Here's how the part is built. I have some questions about the finished solid (model axes, mm). A direction names the side the tool comes from. Give positions to 0.01 mm unless a question says otherwise; leave off trailing zeros. Write each loop counter-clockwise with the first axis right and the second up, starting at its lowest first coordinate (ties: lowest second). Pieces come first, ordered by that corner, then holes. Notation, with made-up numbers: M -37.5,-11.5 L 11.5,-11.5 A15 cw 11.5,-7.5 Z; hole C 89.5,-20.5 d3. An arc over 180 degrees is marked long. Answer as CSV lines item,"result". Start each with the question number.
Q1. For pin 1 (10 mm diameter, centred on x = -1.5, y = 87.5, fed in from +Z); pin 2 (3 mm diameter, centred on x = 29, y = 5.5, fed in from -Z); pin 3 (1.5 mm diameter, centred on x = 7, z = 7.5, fed in from +Y); pin 4 (7.5 mm diameter, centred on y = 43.18, z = 0, fed in from -X), each with a flat end and sliding along its axis, tell me the tip position at first contact or that it passes through.
Q2. Suppose I cut it at B-B (y = 2.5). Write out the boundary of the cut face in (x, z) (3 decimals).
Q3. Thinking about a two-plate mould opening in Z: for faces 1 (the flat face through (-0.812, 56.483, -47.105)), 2 (the cylindrical face through (35.377, 5.151, -7.229)), 3 (the flat face through (-4.318, 60, -50)), which applies, +Z half, -Z half, draft (parallel to the pull), parting line (faces both ways), or undercut?
Q4. Suppose I cut it at A-A (z = 0). Write out the boundary of the cut face in (x, y) (3 decimals), then the cut area to 3 significant figures.
Q5. Suppose I cut it at D-D (z = -33). Write out the boundary of the cut face in (x, y) (3 decimals), then the cut area to 3 significant figures.
Q6. On a 3-axis mill with a long thin cutter (end or side, diameter ignored), from which of +Z, -Z, +X, -X, +Y, -Y can I reach the whole of each face in a straight line? I mean faces 4 (the flat face through (9.906, 42, 38)), 5 (the flat face through (-1, 79, 19.05)), 6 (the flat face through (6, 43, 19.05)), 7 (the flat face through (-0.812, 56.483, 47.105)). Say none if no direction works.
Q7. If I drill on line 1 along X through (y, z) = (-0.5, -42.5); line 2 along X through (y, z) = (58, -47.5); line 3 along Z through (x, y) = (-7, 76.5), over which ranges is the centre line in solid material (lowest first)?
Q8. Suppose I cut it at C-C (x = 0). Write out the boundary of the cut face in (y, z) (3 decimals).
```python
from build123d import *
from build123d.topology import SkipClean

# Parameters (mm, degrees)
SKETCH1_R           = 15.875
SKETCH1_R_2         = 6.35
BOSS_EXTRUDE1_DEPTH = 19.05
BOSS_EXTRUDE2_START = 19.05
SKETCH1_3_R         = 15.875
SKETCH1_3_R_2       = 6.35
BOSS_EXTRUDE2_DEPTH = 38.1
BOSS_EXTRUDE3_START = -19.05
SKETCH1_4_R         = 15.875
SKETCH1_4_R_2       = 6.35
BOSS_EXTRUDE3_DEPTH = 38.1
SKETCH2_W           = 7.112
SKETCH2_H           = 19.812
CUT_EXTRUDE1_DEPTH  = 138.602767
SKETCH4_R           = 6.35
SKETCH4_R_2         = 4.064
CUT_EXTRUDE2_DEPTH  = 123.816814
SKETCH5_R           = 3.175
SKETCH5_R_2         = 5.08
CUT_EXTRUDE3_DEPTH  = 117.109121


with BuildPart() as part:
    # Sketch1 → Boss-Extrude1 (new, symmetric)
    with BuildSketch(Plane.XY):
        Polygon((2.794, 97.536), (-9.906, 72.136), (0, 72.136), (2.794, 72.136), align=None)
        with BuildLine():
            Line((-9.906, 72.136), (-9.906, 12.405111))
            ThreePointArc((-9.906, 12.405111), (-5.24807, 14.982436), (0, 15.875))
            Line((0, 15.875), (0, 72.136))
            Line((0, 72.136), (-9.906, 72.136))
        make_face()
        with BuildLine():
            Line((0, 72.136), (0, 15.875))
            ThreePointArc((0, 15.875), (1.402484, 15.812927), (2.794, 15.627194))
            Line((2.794, 15.627194), (2.794, 72.136))
            Line((2.794, 72.136), (0, 72.136))
        make_face()
        Circle(SKETCH1_R)
        with Locations(Location((0, 0, 0), (0, 0, 180))):
            Circle(SKETCH1_R_2, mode=Mode.SUBTRACT)
        with BuildLine():
            ThreePointArc((12.197952, 10.16), (14.92746, 5.40246), (15.875, 0))
            Line((15.875, 0), (50.8, 0))
            Line((50.8, 0), (50.8, 10.16))
            Line((50.8, 10.16), (12.197952, 10.16))
        make_face()
    extrude(amount=BOSS_EXTRUDE1_DEPTH, both=True)

    # Sketch1<3> → Boss-Extrude2 (add)
    with BuildSketch(Plane.XY.offset(BOSS_EXTRUDE2_START)):
        with BuildLine():
            Line((-9.906, 72.136), (-9.906, 12.405111))
            ThreePointArc((-9.906, 12.405111), (-5.24807, 14.982436), (0, 15.875))
            Line((0, 15.875), (0, 72.136))
            Line((0, 72.136), (-9.906, 72.136))
        make_face()
        Circle(SKETCH1_3_R)
        with Locations(Location((0, 0, 0), (0, 0, 180))):
            Circle(SKETCH1_3_R_2, mode=Mode.SUBTRACT)
        with BuildLine():
            ThreePointArc((2.794, 15.627194), (6.55118, 14.46021), (9.906, 12.405111))
            Line((9.906, 12.405111), (9.906, 72.136))
            Line((9.906, 72.136), (2.794, 72.136))
            Line((2.794, 72.136), (2.794, 15.627194))
        make_face()
        with BuildLine():
            Line((0, 72.136), (0, 15.875))
            ThreePointArc((0, 15.875), (1.402484, 15.812927), (2.794, 15.627194))
            Line((2.794, 15.627194), (2.794, 72.136))
            Line((2.794, 72.136), (0, 72.136))
        make_face()
    extrude(amount=BOSS_EXTRUDE2_DEPTH)

    # Sketch1<4> → Boss-Extrude3 (add)
    with SkipClean():  # the faces are left unmerged after this step: merging them gives an invalid solid
        with BuildSketch(Plane.XY.offset(BOSS_EXTRUDE3_START)):
            with BuildLine():
                ThreePointArc((2.794, 15.627194), (6.55118, 14.46021), (9.906, 12.405111))
                Line((9.906, 12.405111), (9.906, 72.136))
                Line((9.906, 72.136), (2.794, 72.136))
                Line((2.794, 72.136), (2.794, 15.627194))
            make_face()
            with BuildLine():
                Line((-9.906, 72.136), (-9.906, 12.405111))
                ThreePointArc((-9.906, 12.405111), (-5.24807, 14.982436), (0, 15.875))
                Line((0, 15.875), (0, 72.136))
                Line((0, 72.136), (-9.906, 72.136))
            make_face()
            Circle(SKETCH1_4_R)
            with Locations(Location((0, 0, 0), (0, 0, 180))):
                Circle(SKETCH1_4_R_2, mode=Mode.SUBTRACT)
            with BuildLine():
                Line((0, 72.136), (0, 15.875))
                ThreePointArc((0, 15.875), (1.402484, 15.812927), (2.794, 15.627194))
                Line((2.794, 15.627194), (2.794, 72.136))
                Line((2.794, 72.136), (0, 72.136))
            make_face()
        extrude(amount=-BOSS_EXTRUDE3_DEPTH)

    # Sketch2 → Cut-Extrude1 (cut, through all, along a direction that is not the sketch's normal)
    with SkipClean():  # the faces are left unmerged after this step: merging them gives an invalid solid
        with BuildSketch(Plane(origin=(0, 72.136, 0), x_dir=(1, 0, 0), z_dir=(0, 1, 0))):
            with Locations((-0.762, -47.244)):
                Rectangle(SKETCH2_W, SKETCH2_H)
        cut_extrude1 = extrude(amount=-CUT_EXTRUDE1_DEPTH, dir=(0, 0.8483793786580408, -0.5293887322826173), mode=Mode.SUBTRACT)

    # Mirror1: Cut-Extrude1 across plane
    with SkipClean():  # the faces are left unmerged after this step: merging them gives an invalid solid
        add(cut_extrude1.mirror(Plane.XY), mode=Mode.SUBTRACT)

    # Sketch4 → Cut-Extrude2 (cut, through all)
    with SkipClean():  # the faces are left unmerged after this step: merging them gives an invalid solid
        with BuildSketch(Plane(origin=(2.794, 0, 0), x_dir=(0, 0, -1), z_dir=(1, 0, 0))):
            with BuildLine():
                Line((-6.35, 97.536), (-6.35, 72.136))
                ThreePointArc((-6.35, 72.136), (0, 78.486), (6.35, 72.136))
                Line((6.35, 72.136), (6.35, 97.536))
                Line((6.35, 97.536), (-6.35, 97.536))
            make_face()
            with Locations((0, 72.136)):
                Circle(SKETCH4_R)
            with Locations((0, 43.18)):
                Circle(SKETCH4_R_2)
        extrude(amount=-CUT_EXTRUDE2_DEPTH, mode=Mode.SUBTRACT)

    # Sketch5 → Cut-Extrude3 (cut, through all)
    with SkipClean():  # the faces are left unmerged after this step: merging them gives an invalid solid
        with BuildSketch(Plane(origin=(0, 10.16, 0), x_dir=(1, 0, 0), z_dir=(0, 1, 0))):
            with Locations(Location((37.084, -9.906, 0), (0, 0, 180))):
                Circle(SKETCH5_R)
            with Locations(Location((37.084, 9.906, 0), (0, 0, 180))):
                Circle(SKETCH5_R)
            with Locations((50.8, 0)):
                Circle(SKETCH5_R_2)
        extrude(amount=-CUT_EXTRUDE3_DEPTH, mode=Mode.SUBTRACT)


solid = part.part
```
Resolved:
1,pin 1,"z = 19.05"
1,pin 2,"z = -19.05"
1,pin 3,"y = 14.59"
1,pin 4,"through"
2,outline,"M -15.677,-57.15 L -5.837,-57.15 L -5.837,57.15 L -15.677,57.15 Z; M 5.837,-57.15 L 15.677,-57.15 L 15.677,-19.05 L 50.8,-19.05 L 50.8,-5.08 A5.08 cw 50.8,5.08 L 50.8,19.05 L 15.677,19.05 L 15.677,57.15 L 5.837,57.15 Z; hole C 37.084,-9.906 d6.35; hole C 37.084,9.906 d6.35"
3,face 1,"-Z half"
3,face 2,"undercut"
3,face 3,"draft"
4,outline,"M -9.906,12.405 A15.875 ccw long 15.875,0 L 45.72,0 L 45.72,10.16 L 12.198,10.16 A15.875 ccw 2.794,15.627 L 2.794,39.116 L -9.906,39.116 Z; M -9.906,47.244 L 2.794,47.244 L 2.794,65.786 L -9.906,65.786 Z; hole C 0,0 d12.7"
4,area,"1,520 mm^2"
5,outline,"M -9.906,12.405 A15.875 ccw long 9.906,12.405 L 9.906,72.136 L -9.906,72.136 Z; hole C 0,0 d12.7"
5,area,"1,800 mm^2"
6,face 4,"+Z, -Z, +X, +Y"
6,face 5,"+Z, +X, -X, +Y"
6,face 6,"+X, +Y"
6,face 7,"+Z, +Y"
7,line 1,"-15.87 to -6.33, 6.33 to 15.87"
7,line 2,"-9.91 to -4.32, 2.79 to 9.91"
7,line 3,"-19.05 to -6.35, 6.35 to 19.05"
8,outline,"M -15.875,-57.15 L -6.35,-57.15 L -6.35,57.15 L -15.875,57.15 Z; M 6.35,-57.15 L 40.386,-57.15 L 72.136,-37.338 L 72.136,-19.05 L 91.948,-19.05 L 91.948,-6.35 L 72.136,-6.35 A6.35 cw 72.136,6.35 L 91.948,6.35 L 91.948,19.05 L 72.136,19.05 L 72.136,37.338 L 40.386,57.15 L 6.35,57.15 Z; hole C 43.18,0 d8.128"
